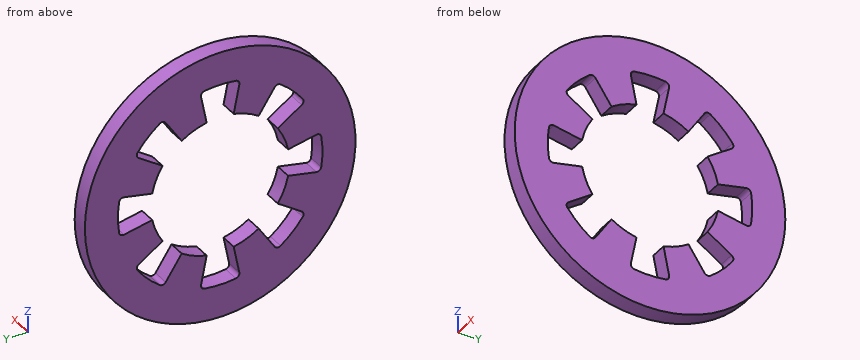
Autodesk Inventor part; units mm, degrees
ref_plane "Work Plane1" through (0, 0, 0) normal (0, 1, 0) x (1, 0, 0)
ref_plane "YZ Plane" through (0, 0, 0) normal (1, 0, 0) x (0, 1, 0)
ref_plane "XZ Plane" through (0, 0, 0) normal (0, 1, 0) x (-1, 0, 0)
sketch "Sketch1" plane through (0, 0, 0) normal (1, 0, 0) x (0, 1, 0)
  circle A0 centre (0, 0) radius 4.8387
  circle A1 centre (0, 0) radius 2.4765
  dimension "d0" = 9.6774
  dimension "d1" = 4.953
extrude "Body" add sketch "Sketch1" along normal blind 0.6096
sketch "Sketch2" plane through (0, 0, 0) normal (-1, 0, 0) x (0, 0, 1)
  circle A0 centre (0, 0) radius 2.4765
  circle A1 centre (0, 0) radius 4.8387
  arc A2 (0.7136, 3.5873) -> (-0.7136, 3.5873) centre (0, 0) ccw
  line L0 (-0.4831, 2.4289) -> (-0.7136, 3.5873)
  line L1 (0, 0) -> (0, 3.6576) construction
  line L2 (0.4831, 2.4289) -> (0.7136, 3.5873)
  line L3 (-0.4831, 2.4289) -> (0, 0) construction
  line L4 (0.4831, 2.4289) -> (0, 0) construction
  dimension "d4" = 7.3152
  dimension "d5" = 11.25
extrude "Cut" cut sketch "Sketch2" against normal blind 0.6096 contours A0 L0 A2 L2
fillet "Fillet1" radius 0.1486 2 edges at (0.3048, 3.5873, 0.7136) (0.3048, 3.5873, -0.7136)
pattern_circular "Cuts" count 8 over 360 about axis through (-10, 0, 0) along (1, 0, 0) of "Cut", "Fillet1"
ref_plane "Work Plane1" through (0, 0, 0) normal (0, 1, 0) x (1, 0, 0)
equation "\"d0\" = SD2"
equation "\"d1\" = SD1"
equation "\"d2\" = SD"
equation "\"d4\" = 0.5 * SD2 + 0.5 * SD1"
equation "\"d6\" = SD"
equation "\"d8\" = 0.03 * SD1"
equation "\"SD1\" = 4.953"
equation "\"SD2\" = 9.6774"
equation "\"SD\" = 0.6096"
equation "\"NND\" = 4.826"
properties part number "ASME B18.21.1 - No. 10. Carbon Steel" material "Steel, Mild"
Design review of the part built by this model. Coordinates are the model's own, in mm. Give positions to 0.01 mm unless a question says otherwise; leave off trailing zeros. Write each loop counter-clockwise with the first axis right and the second up, starting at its lowest first coordinate (ties: lowest second). Pieces come first, ordered by that corner, then holes. Notation, with made-up numbers: M -4,-3.5 L 53,-3.5 A10 cw 53,9.5 Z; hole C 33,27.25 d3. An arc over 180 degrees is marked long. Return JSON: item names as keys, results as strings. Group by question number.
Item 1: Take a section at A-A (y = 0). Give the boundary of the cut face in (x, z), plus the area to 3 significant figures.
Item 2: Take a section at C-C (y = 4). Give the boundary of the cut face in (x, z).
Item 3: Clearance check with a flat-ended pin moving along its axis: pin 1 Ø5 at (y, z) = (-3, 1) entering from -X. State where the tip first meets the part, or that it passes through.
Item 4: Wall thickness on line 1 along Y through (x, z) = (0.4, 2.75); line 2 along Z through (x, y) = (0.35, 0); line 3 along Y through (x, z) = (0.5, -1.5): over which ranges is each line inside the solid? List them lowest first.
Return value:
{
 "1": {"outline": "M 0,-4.84 L 0.61,-4.84 L 0.61,-3.66 L 0,-3.66 Z; M 0,3.66 L 0.61,3.66 L 0.61,4.84 L 0,4.84 Z", "area": "1.44 mm2"},
 "2": {"outline": "M 0,-2.72 L 0.61,-2.72 L 0.61,2.72 L 0,2.72 Z"},
 "3": {"pin 1": "stops at x = 0"},
 "4": {"line 1": "y = -3.98 to -2.41, -1.84 to -0.55, 0.55 to 1.84, 2.41 to 3.98", "line 2": "z = -4.84 to -3.66, 3.66 to 4.84", "line 3": "y = -4.6 to -2.24, 2.24 to 4.6"}
}
